Verification items for the finished model (mm, model axes). Give positions to 0.01 mm unless a question says otherwise; leave off trailing zeros. Loops run counter-clockwise (first coordinate to the right, second up) from the corner with the lowest first, then second, coordinate; pieces in that order, holes last. Notation, with made-up numbers: M 28,68 L 54,68 A28 ccw 54,95 Z; hole C -36,50 d9. An arc over 180 degrees is marked long. Answer in a Markdown table with one row per item.
```python
from build123d import *

# Parameters (mm, degrees)
BOSS_EXTRUDE1_DEPTH = 4
SKETCH4_W           = 8
SKETCH4_H           = 1.8
CUT_EXTRUDE2_DEPTH  = 2
FILLET1_R           = 1
FILLET2_R           = 0.2


with BuildPart() as part:
    # Sketch1 → Boss-Extrude1 (new body)
    with BuildSketch(Plane.XY):
        with BuildLine():
            Line((0, 0), (10, 0))
            ThreePointArc((10, 0), (8.189187828, 1.718754897), (6.384188985, 3.443613817))
            ThreePointArc((6.384188985, 3.443613817), (4.997832528, 3.999998826), (3.612685275, 3.440610236))
            ThreePointArc((3.612685275, 3.440610236), (1.811114467, 1.715294636), (0, 0))
        make_face()
    extrude(amount=BOSS_EXTRUDE1_DEPTH)

    # Cut-Extrude1: read off the stored shape, not the designer's step
    # Cut-Extrude1: loft between two sections, ruled curve by curve
    cut_extrude1_from = [
        Edge.make_line((3.279743704, 2.191579296, 0.102519741), (3.279743704, 2.41730023, 0.102519741)),
        Edge.make_line((3.279743704, 2.41730023, 0.102519741), (6.720256296, 2.41730023, 0.102519741)),
        Edge.make_line((6.720256296, 2.41730023, 0.102519741), (6.720256296, 2.191579296, 0.102519741)),
        Edge.make_line((6.720256296, 2.191579296, 0.102519741), (3.279743704, 2.191579296, 0.102519741)),
    ]
    cut_extrude1_to = [
        Edge.make_line((3, 1, 4), (3, 1.8, 4)),
        Edge.make_line((3, 1.8, 4), (7, 1.8, 4)),
        Edge.make_line((7, 1.8, 4), (7, 1, 4)),
        Edge.make_line((7, 1, 4), (3, 1, 4)),
    ]
    cut_extrude1 = Solid(Shell([*[Face.make_surface_from_curves(cut_extrude1_from[k], cut_extrude1_to[k]) for k in range(4)], Face(Wire(cut_extrude1_from)), Face(Wire(cut_extrude1_to))]))
    add(cut_extrude1, mode=Mode.SUBTRACT)

    # Sketch4 → Cut-Extrude2 (cut)
    with BuildSketch(Plane.XY.offset(4)):
        with Locations((4.997832528, 0.9)):
            Rectangle(SKETCH4_W, SKETCH4_H)
    extrude(amount=-CUT_EXTRUDE2_DEPTH, mode=Mode.SUBTRACT)

    # Fillet1
    fillet1_edges = [part.edges().sort_by_distance(p)[0] for p in [
        (0, 0, 2),
        (10, 0, 2),
    ]]
    fillet(fillet1_edges, radius=FILLET1_R)

    # Fillet2
    fillet2_edges = [part.edges().sort_by_distance(p)[0] for p in [
        (1.900031879, 1.8, 3),
        (8.103893685, 1.8, 3),
    ]]
    fillet(fillet2_edges, radius=FILLET2_R)


solid = part.part
```
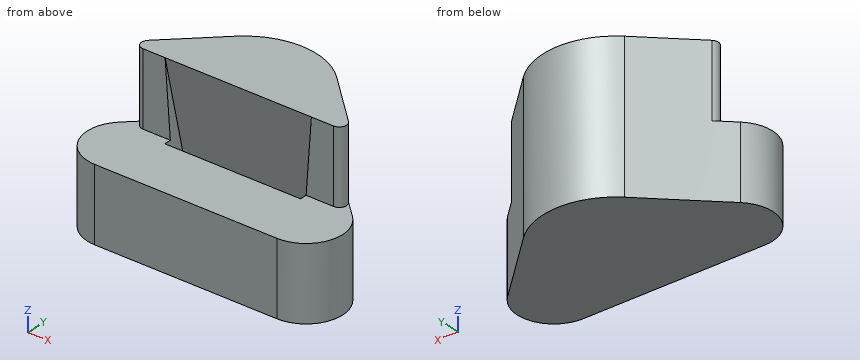
Item 1: Sectioned sample at A-A (y = 3.3). Record the cut outline in (x, z), and give its area (3 significant figures).
Reported:
| item | result |
|---|---|
| outline | M 3.47,0 L 6.53,0 L 6.53,4 L 3.47,4 Z |
| area | 12.3 mm^2 |
Item 2: Sectioned sample at B-B (y = 0.25). Record the cut outline in (x, z), and give its area (3 significant figures).
Reported:
| item | result |
|---|---|
| outline | M 1.85,0 L 8.16,0 L 8.16,2 L 1.85,2 Z |
| area | 12.6 mm^2 |
Item 3: Scan lines: L1, parallel to Y at x = 6.5, z = 0.35; L2, parallel to Z at x = 3.5, y = 1.55; L3, parallel to Y at x = 5, z = 1.2. Record each from-to range of solid material in increasing order. Write a range as [from, to].
Reported:
| item | result |
|---|---|
| L1 | y = [0, 2.12], [2.38, 3.33] |
| L2 | z = [0, 2] |
| L3 | y = [0, 1.86], [2.24, 4] |
Item 4: Go/stop test with flat-tipped pins: pin 1 (0.8 mm diameter, centred on x = 7, z = 3, fed in from -Y); pin 2 (2 mm diameter, centred on x = 4, y = 1, fed in from +Z). Record where each tip stops, or that it passes through.
Reported:
| item | result |
|---|---|
| pin 1 | stops at y = 1.8 |
| pin 2 | stops at z = 4 |
